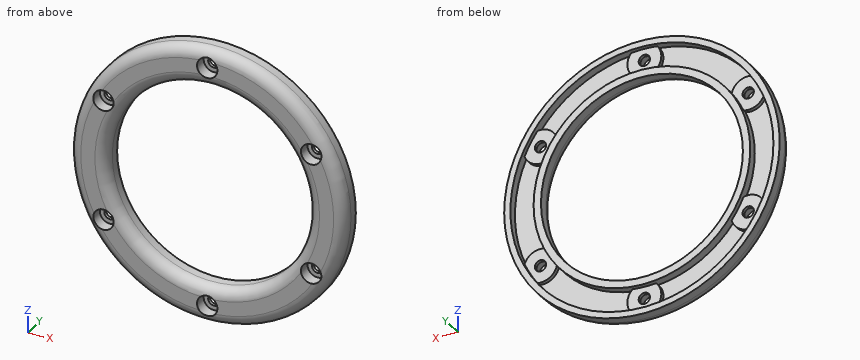
```python
from build123d import *

# Parameters (mm, degrees)
F0_R     = 30.9245
F0_R_2   = 22.6695
F1_DEPTH = 4.572
F2_R     = 29.5275
F2_R_2   = 24.3205
F3_DEPTH = 1.905
F4_R     = 3.81
F5_DEPTH = 0.889
F6_R     = 1.27
F7_DEPTH = 3.557
F8_R     = 2.286
F9_DEPTH = 2.794


# Not quite as in the source:
# - a fillet or chamfer that OpenCascade refuses, or shapes differently, is made with other operations: its cross-section is extruded or revolved along the edge and cut away or added


with BuildPart() as f1:
    # F0 (on Front) → F1 (new body)
    with BuildSketch(Plane.XZ):
        Circle(F0_R)
        Circle(F0_R_2, mode=Mode.SUBTRACT)
    extrude(amount=F1_DEPTH)

    # F2 (on face) → F3 (cut)
    with BuildSketch(Plane(origin=(0, 0, 0), x_dir=(-1, 0, 0), z_dir=(0, 1, 0))):
        Circle(F2_R)
        Circle(F2_R_2, mode=Mode.SUBTRACT)
    extrude(amount=-F3_DEPTH, mode=Mode.SUBTRACT)

    # F4 (on face) → F5 (join)
    with BuildSketch(Plane(origin=(0, -1.905, 0), x_dir=(-1, 0, 0), z_dir=(0, 1, 0))):
        with Locations((0, 26.924)):
            Circle(F4_R)
        with Locations((-23.3168679715, 13.462)):
            Circle(F4_R)
        with Locations((-23.3168679715, -13.462)):
            Circle(F4_R)
        with Locations((0, -26.924)):
            Circle(F4_R)
        with Locations((23.3168679715, -13.462)):
            Circle(F4_R)
        with Locations((23.3168679715, 13.462)):
            Circle(F4_R)
    extrude(amount=F5_DEPTH)

    # F6 (on face) → F7 (cut, through all)
    with BuildSketch(Plane(origin=(0, -1.016, 0), x_dir=(-1, 0, 0), z_dir=(0, 1, 0))):
        with Locations((0, 26.924)):
            Circle(F6_R)
        with Locations((-23.3168679715, 13.462)):
            Circle(F6_R)
        with Locations((-23.3168679715, -13.462)):
            Circle(F6_R)
        with Locations((0, -26.924)):
            Circle(F6_R)
        with Locations((23.3168679715, -13.462)):
            Circle(F6_R)
        with Locations((23.3168679715, 13.462)):
            Circle(F6_R)
    extrude(amount=-F7_DEPTH, mode=Mode.SUBTRACT)

    # F8 (on face) → F9 (cut)
    with BuildSketch(Plane.XZ.offset(4.572)):
        with Locations((0, 26.924)):
            Circle(F8_R)
        with Locations((-23.3168679715, 13.462)):
            Circle(F8_R)
        with Locations((-23.3168679715, -13.462)):
            Circle(F8_R)
        with Locations((0, -26.924)):
            Circle(F8_R)
        with Locations((23.3168679715, -13.462)):
            Circle(F8_R)
        with Locations((23.3168679715, 13.462)):
            Circle(F8_R)
    extrude(amount=-F9_DEPTH, mode=Mode.SUBTRACT)

    # F10: fillet of radius 2.54 on 2 edges, made by hand

    # F10_s1 → F10_t2 (revolve, cut)
    with BuildSketch(Plane.XY):
        with BuildLine():
            ThreePointArc((30.9245, -2.032), (30.1805512242, -3.8280512242), (28.3845, -4.572))
            Line((28.3845, -4.572), (30.9245, -4.572))
            Line((30.9245, -4.572), (30.9245, -2.032))
        make_face()
    revolve(axis=Axis((0, -4.572, 0), (0, -1, 0)), mode=Mode.SUBTRACT)

    # F10_s3 → F10_t4 (revolve, cut)
    with BuildSketch(Plane.XY):
        with BuildLine():
            ThreePointArc((25.2095, -4.572), (23.4134487758, -3.8280512242), (22.6695, -2.032))
            Line((22.6695, -2.032), (22.6695, -4.572))
            Line((22.6695, -4.572), (25.2095, -4.572))
        make_face()
    revolve(axis=Axis((0, -4.572, 0), (0, -1, 0)), mode=Mode.SUBTRACT)


solid = f1.part
```
CAD build for the part. Positions are in the model's coordinates, mm. Round coordinates to 2 decimals unless told otherwise and drop trailing zeros. Loops run counter-clockwise (first coordinate to the right, second up) from the corner with the lowest first, then second, coordinate; pieces in that order, holes last. Notation, with made-up numbers: M -17.75,73.5 L -7.75,73.5 A28 ccw -7.75,108.5 Z; hole C -13.5,-19 d9. An arc over 180 degrees is marked long. Return JSON: item names as keys, results as strings. Group by question number.
(1) Saw through at B-B, the plane x = 0. Give the number of separate pieces and of enclosed holes in the cut face, and give its area (3 significant figures).
(2) Saw through at A-A, the plane z = 0. List the corners of the cut face in (x, y) (1 decimal), and give its area (3 significant figures).
(3) Drop flat-ended pins along their axis: P1, Ø1.4, axis at x = 23.5, z = -13.5, coming from the -Y side; P2, Ø3.5, axis at x = 23.32, z = -13.46, coming from the +Y side; P3, Ø1.4, axis at x = -23.5, z = 12.5, coming from the -Y side; P4, Ø2, axis at y = -1.5, z = 16.5, coming from the -X side. Give the stop position or say it passes through.
(4) Wall check: probe 1 along Z at (x, y) = (0, -1.15); probe 2 along X at (y, z) = (-0.65, -20); probe 3 along Z at (x, y) = (1, -1.25). Give the ranges that are in metal, low to high. Write a range as [from, to].
Answer list:
{
 "1": {"separate pieces": "4", "enclosed holes": "0", "area": "30.0 mm2"},
 "2": {"outline": "M -30.9,-2 A2.5 ccw -28.4,-4.6 L -25.2,-4.6 A2.5 ccw -22.7,-2 L -22.7,0 L -24.3,0 L -24.3,-1.9 L -29.5,-1.9 L -29.5,0 L -30.9,0 Z; M 22.7,-2 A2.5 ccw 25.2,-4.6 L 28.4,-4.6 A2.5 ccw 30.9,-2 L 30.9,0 L 29.5,0 L 29.5,-1.9 L 24.3,-1.9 L 24.3,0 L 22.7,0 Z", "area": "50.1 mm2"},
 "3": {"P1": "through", "P2": "y = -1.02", "P3": "y = -1.78", "P4": "x = -26.76"},
 "4": {"probe 1": "[-30.92, -28.19], [-25.65, -22.67], [22.67, 25.65], [28.19, 30.92]", "probe 2": "[-23.59, -21.72], [-13.84, -10.67], [10.67, 13.84], [21.72, 23.59]", "probe 3": "[-30.91, -27.71], [-26.14, -22.65], [22.65, 26.14], [27.71, 30.91]"}
}
